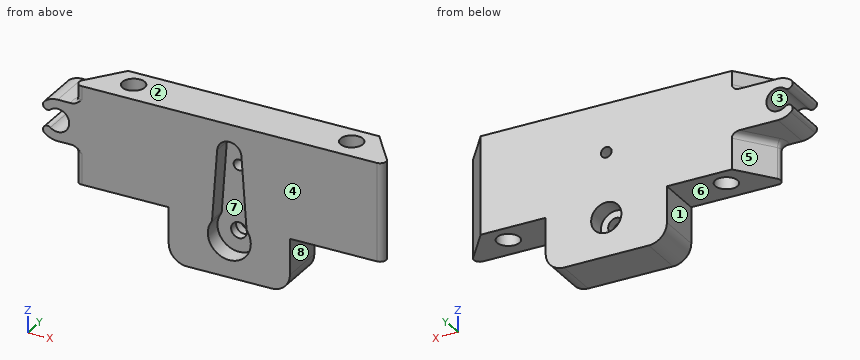
```python
from build123d import *

# Parameters (mm, degrees)
BOSS_EXTRUDE1_DEPTH      = 4.425
BOSS_EXTRUDE1_DEPTH_BACK = 2.9
CUT_EXTRUDE1_DEPTH       = 34.079090828
SKETCH6_R                = 1.3
CUT_EXTRUDE2_DEPTH       = 34.590195742
SKETCH7_R                = 2.5
CUT_EXTRUDE3_DEPTH       = 2.925
SKETCH8_R                = 0.875
CUT_EXTRUDE4_DEPTH       = 34.079090828
SKETCH9_R                = 1.85
CUT_EXTRUDE5_DEPTH       = 32.712487288
CUT_EXTRUDE6_DEPTH       = 38.074873567
FILLET1_R                = 1
FILLET2_R                = 3
BOSS_EXTRUDE2_DEPTH      = 7.325
FILLET3_R                = 1


with BuildPart() as part:
    # Sketch4 → Boss-Extrude1 (new, two sides: drawn at the far end of the back side and taken through both)
    with BuildSketch(Plane(origin=(0, 0, 0), x_dir=(1, 0, 0), z_dir=(0, 1, 0)).offset(-BOSS_EXTRUDE1_DEPTH_BACK)):
        Polygon((-26.925, -2.54), (-10.000436291, -2.54), (-10.000436291, 6.4), (10.000436291, 6.4), (10.000436291, -2.54), (26.925, -2.54), (26.925, -18.7), (-26.925, -18.7), align=None)
    extrude(amount=BOSS_EXTRUDE1_DEPTH + BOSS_EXTRUDE1_DEPTH_BACK)

    # Sketch5 → Cut-Extrude1 (cut, through all)
    with BuildSketch(Plane(origin=(0, 0, 0), x_dir=(1, 0, 0), z_dir=(0, 1, 0))):
        with BuildLine():
            Line((2.004851846, -13.98376743), (2.839866559, -2.339399967))
            ThreePointArc((2.839866559, -2.339399967), (2.881992781, -2.129359863), (2.975294921, -1.936522692))
            ThreePointArc((2.975294921, -1.936522692), (0, 3.55), (-2.975294921, -1.936522692))
            ThreePointArc((-2.975294921, -1.936522692), (-2.881992781, -2.129359863), (-2.839866559, -2.339399967))
            Line((-2.839866559, -2.339399967), (-2.004851846, -13.98376743))
            ThreePointArc((-2.004851846, -13.98376743), (0, -15.85), (2.004851846, -13.98376743))
        make_face()
    extrude(amount=-CUT_EXTRUDE1_DEPTH, mode=Mode.SUBTRACT)

    # Sketch6 → Cut-Extrude2 (cut, through all)
    with BuildSketch(Plane(origin=(0, 4.425, 0), x_dir=(1, 0, 0), z_dir=(0, 1, 0))):
        with Locations(Location((0, 0, 0), (0, 0, 270))):
            Circle(SKETCH6_R)
    extrude(amount=-CUT_EXTRUDE2_DEPTH, mode=Mode.SUBTRACT)

    # Sketch7 → Cut-Extrude3 (cut)
    with BuildSketch(Plane(origin=(0, 4.425, 0), x_dir=(1, 0, 0), z_dir=(0, 1, 0))):
        with Locations(Location((0, 0, 0), (0, 0, 270))):
            Circle(SKETCH7_R)
    extrude(amount=-CUT_EXTRUDE3_DEPTH, mode=Mode.SUBTRACT)

    # Sketch8 → Cut-Extrude4 (cut, through all)
    with BuildSketch(Plane.XZ):
        with Locations(Location((0, 10.7, 0), (0, 0, 270))):
            Circle(SKETCH8_R)
    extrude(amount=-CUT_EXTRUDE4_DEPTH, mode=Mode.SUBTRACT)

    # Sketch9 → Cut-Extrude5 (cut, through all)
    with BuildSketch(Plane(origin=(0, 0, 2.54), x_dir=(-1, 0, 0), z_dir=(0, 0, -1))):
        with Locations((18, 1.1)):
            Circle(SKETCH9_R)
        with Locations((-18, 1.1)):
            Circle(SKETCH9_R)
    extrude(amount=-CUT_EXTRUDE5_DEPTH, mode=Mode.SUBTRACT)

    # Sketch11 → Cut-Extrude6 (cut, through all)
    with BuildSketch(Plane.XY.offset(18.7)):
        Polygon((-20.723540873, 4.425), (-26.372623028, -2.9), (-26.925, -2.9), (-26.925, 4.425), align=None)
        Polygon((20.723540873, 4.425), (26.925, 4.425), (26.925, -2.9), (26.372623028, -2.9), align=None)
    extrude(amount=-CUT_EXTRUDE6_DEPTH, mode=Mode.SUBTRACT)

    # Fillet1
    fillet1_edges = [part.edges().sort_by_distance(p)[0] for p in [
        (26.372623028, -2.9, 10.62),
        (-26.372623028, -2.9, 10.62),
    ]]
    fillet(fillet1_edges, radius=FILLET1_R)

    # Fillet2
    fillet2_edges = [part.edges().sort_by_distance(p)[0] for p in [
        (-10.000436291, 0.7625, -6.4),
        (10.000436291, 0.7625, -6.4),
    ]]
    fillet(fillet2_edges, radius=FILLET2_R)

    # Sketch14 → Boss-Extrude2 (add, through all)
    with BuildSketch(Plane(origin=(0, 4.425, 0), x_dir=(1, 0, 0), z_dir=(0, 1, 0))):
        with BuildLine():
            Line((-20.723540873, -8.65), (-28.322297461, -8.65))
            ThreePointArc((-28.322297461, -8.65), (-29.466272656, -8.848231621), (-30.476852522, -9.419811321))
            ThreePointArc((-30.476852522, -9.419811321), (-30.581771703, -10.475269499), (-29.526313525, -10.580188679))
            ThreePointArc((-29.526313525, -10.580188679), (-26.422297461, -12.05), (-29.526313525, -13.519811321))
            ThreePointArc((-29.526313525, -13.519811321), (-30.581771703, -13.624730501), (-30.476852522, -14.680188679))
            ThreePointArc((-30.476852522, -14.680188679), (-29.466272656, -15.251768379), (-28.322297461, -15.45))
            Line((-28.322297461, -15.45), (-20.723540873, -15.45))
            Line((-20.723540873, -15.45), (-20.723540873, -8.65))
        make_face()
    extrude(amount=-BOSS_EXTRUDE2_DEPTH)

    # Fillet3
    # the kernel refuses this fillet: 1 mm, written as the material it adds along each edge
    with BuildSketch(Plane(origin=(-24.338579866, -1.9, 8.65), x_dir=(0.5968522081551058, 0.8023511959362772, 0), z_dir=(-0.8023511959362772, 0.5968522081551058, 0))) as fillet3_piece_1_section:
        with BuildLine():
            CenterArc((1 + FILLET3_R, FILLET3_R), FILLET3_R, 180, 90)
            Line((1, FILLET3_R), (1, 0))
            Line((1, 0), (1 + FILLET3_R, 0))
        make_face()
    fillet3_piece_1 = revolve(axis=Axis((-24.338579866, -1.9, 8.65), (0, 0, -1)), revolution_arc=270.994831495, mode=Mode.PRIVATE)
    fillet3_piece_1 = split(fillet3_piece_1, bisect_by=Plane(origin=(-25.318581696, -2.9, 8.393059432), z_dir=(0, 1, 0)), keep=Keep.TOP, mode=Mode.PRIVATE)
    add(fillet3_piece_1)
    with BuildSketch(Plane(origin=(-24.338579866, -1.9, 15.45), x_dir=(0.5968522081551029, 0.8023511959362795, 0), z_dir=(-0.8023511959362795, 0.5968522081551029, 0))) as fillet3_piece_2_section:
        with BuildLine():
            CenterArc((1 + FILLET3_R, -FILLET3_R), FILLET3_R, 90, 90)
            Line((1 + FILLET3_R, 0), (1, 0))
            Line((1, 0), (1, -FILLET3_R))
        make_face()
    fillet3_piece_2 = revolve(axis=Axis((-24.338579866, -1.9, 15.45), (0, 0, -1)), revolution_arc=270.994831495, mode=Mode.PRIVATE)
    fillet3_piece_2 = split(fillet3_piece_2, bisect_by=Plane(origin=(-25.318581739, -2.9, 15.706940487), z_dir=(0, 1, 0)), keep=Keep.TOP, mode=Mode.PRIVATE)
    add(fillet3_piece_2)
    with BuildSketch(Plane(origin=(-25.130447445, -1.289307166, 15.45), x_dir=(0, 0, 1), z_dir=(0.6106928339923638, 0.7918675788983757, 0))) as fillet3_piece_3_section:
        with BuildLine():
            CenterArc((FILLET3_R, -FILLET3_R), FILLET3_R, 90, 90)
            Line((0, -FILLET3_R), (0, 0))
            Line((0, 0), (FILLET3_R, 0))
        make_face()
    fillet3_piece_3 = extrude(amount=9.716240844, mode=Mode.PRIVATE)
    fillet3_piece_3 = split(fillet3_piece_3, bisect_by=Plane(origin=(-23.152517153, 4.425, 15.675632439), z_dir=(0, -1, 0)), keep=Keep.TOP, mode=Mode.PRIVATE)
    add(fillet3_piece_3)
    with BuildSketch(Plane(origin=(-19.196808788, 6.404668947, 8.65), x_dir=(0, 0, -1), z_dir=(-0.6106928339923638, -0.7918675788983757, 0))) as fillet3_piece_4_section:
        with BuildLine():
            CenterArc((FILLET3_R, -FILLET3_R), FILLET3_R, 90, 90)
            Line((0, -FILLET3_R), (0, 0))
            Line((0, 0), (FILLET3_R, 0))
        make_face()
    fillet3_piece_4 = extrude(amount=9.716240844, mode=Mode.PRIVATE)
    fillet3_piece_4 = split(fillet3_piece_4, bisect_by=Plane(origin=(-23.152517153, 4.425, 8.424367561), z_dir=(0, -1, 0)), keep=Keep.TOP, mode=Mode.PRIVATE)
    add(fillet3_piece_4)


solid = part.part
```
Geometry check sheet. Reference: the model listing, model coordinates, mm. Face numbers are marked on the shaded views. A direction names the side the tool comes from. Round coordinates to 2 decimals unless told otherwise and drop trailing zeros. Order: outer loops, then holes, each group sorted by start corner. A loop starts at its lowest first (then second) coordinate and runs counter-clockwise, first axis right, second up. Notation, with made-up numbers: (21.5, 17.25) -> (46.5, 17.25) arc R33 cw to (46.5, 46.25) -> close; hole circle Ø9 at (7, 32). An arc over 180 degrees is marked (long way). Return JSON: item names as keys, results as strings. Group by question number.
Q1. Gauge pin test, flat ends, axial feed: pin 1 (2.5 mm diameter, centred on x = -0.5, z = 0.5, fed in from +Y); pin 2 (2 mm diameter, centred on x = -18, y = 1.1, fed in from +Z); pin 3 (1.8 mm diameter, centred on y = 0.5, z = -0.5, fed in from -X); pin 4 (3.5 mm diameter, centred on x = 21, y = 1, fed in from -Z). Record the tip position at first contact, or that the pin passes through.
Q2. Material ranges on probe 1 along X at (y, z) = (4, -1.5); probe 2 along X at (y, z) = (1.5, 17.5); probe 3 along X at (y, z) = (-1.05, 0), recorded low to high. Write a range as from..to.
Q3. Tool access check on the marked faces 4, 5, 6, 7 and 8. Record the directions out of +Z, -Z, +X, -X, +Y, -Y that give a thin tool (end or side, any length) a straight path to the whole face; none if there is none.
Q4. Section check B-B, the plane z = 0. Record the boundary of the cut face in (x, y) (3 decimals), plus the area to 3 significant figures.
Q5. Section check C-C, the plane y = 2. Count the separate pieces of the cut face and the enclosed holes in it, plus the area to 3 significant figures.
Q6. Release check for a two-part mould opening along X. For the marked faces 1, 2 and 3 record: released by +X, released by -X, zero draft, split by the parting line, or undercut.
Q7. Section check D-D, the plane z = 6.75. Record the boundary of the cut face in (x, y) (3 decimals).
Q8. Section check A-A, the plane x = 18. Record the boundary of the cut face in (y, z) (3 decimals).
Numbers:
{
 "1": {"pin 1": "y = 1.5", "pin 2": "through", "pin 3": "x = -10", "pin 4": "z = 2.54"},
 "2": {"probe 1": "-10..-2, 2..10", "probe 2": "-22.98..-19.81, -16.19..16.19, 19.81..22.98", "probe 3": "-10..-3.55, 3.55..10"},
 "3": {"face 4": "+Z, -Z, +X, -X, -Y", "face 5": "-Z, -X, +Y", "face 6": "-Z, -X, +Y, -Y", "face 7": "-Y", "face 8": "-Z, +X, +Y, -Y"},
 "4": {"outline": "(-10, -2.9) -> (-3.55, -2.9) -> (-3.55, 0) -> (-1.3, 0) -> (-1.3, 1.5) -> (-2.5, 1.5) -> (-2.5, 4.425) -> (-10, 4.425) -> close; (1.3, 0) -> (3.55, 0) -> (3.55, -2.9) -> (10, -2.9) -> (10, 4.425) -> (2.5, 4.425) -> (2.5, 1.5) -> (1.3, 1.5) -> close", "area": "107 mm^2"},
 "5": {"separate pieces": "3", "enclosed holes": "2", "area": "820 mm^2"},
 "6": {"face 1": "released by -X", "face 2": "zero draft", "face 3": "undercut"},
 "7": {"outline": "(-25.13, -1.289) arc R1 ccw to (-24.339, -2.9) -> (-2.524, -2.9) -> (-2.524, 0) -> (2.524, 0) -> (2.524, -2.9) -> (24.339, -2.9) arc R1 ccw to (25.13, -1.289) -> (20.724, 4.425) -> (-20.724, 4.425) -> close; hole circle Ø3.7 at (-18, 1.1); hole circle Ø3.7 at (18, 1.1)"},
 "8": {"outline": "(-2.9, 2.54) -> (-0.75, 2.54) -> (-0.75, 18.7) -> (-2.9, 18.7) -> close; (2.95, 2.54) -> (4.425, 2.54) -> (4.425, 18.7) -> (2.95, 18.7) -> close"}
}
